Design review of the part built by this model. Coordinates are the model's own, in mm. Give positions to 0.01 mm unless a question says otherwise; leave off trailing zeros. Loops run counter-clockwise (first coordinate to the right, second up) from the corner with the lowest first, then second, coordinate; pieces in that order, holes last. Notation, with made-up numbers: (26, 40.5) -> (42, 40.5) arc R28 ccw to (42, 67.5) -> close; hole circle Ø1 at (76, 62.5). An arc over 180 degrees is marked (long way). Use CSV: the item, a comma, the result in double quotes. Start each with the question number.
Item 1: We need section A-A (x = 279). State the section outline as (y, z) points.
Item 2: Wall thickness on line 1 along X through (y, z) = (-1.25, 0); line 2 along Z through (x, y) = (138.5, 0.9); line 3 along Z through (x, y) = (308.5, 1.7): over which ranges is each line inside the solid? List them lowest first. Write a range as from..to.
Item 3: Clearance check with flat-ended pins moving along their axes: pin 1 (0.6 mm diameter, centred on x = 205, y = 2.5, fed in from +Z); pin 2 (2.5 mm diameter, centred on x = 336.35, z = 0, fed in from -Y); pin 3 (2.5 mm diameter, centred on x = 138, z = -1.5, fed in from +Y). State where each tip first meets the part, or that it passes through.
from build123d import *

# Parameters (mm, degrees)
BOSS_EXTRUDE1_DEPTH = 350
SKETCH6_R           = 1.6
CUT_EXTRUDE1_DEPTH  = 351.117823025


with BuildPart() as part:
    # Sketch5 → Boss-Extrude1 (new body)
    with BuildSketch(Plane(origin=(0, 0, 0), x_dir=(0, 0, -1), z_dir=(1, 0, 0))):
        with BuildLine():
            Line((-8.499999996, -2.75), (8.499999996, -2.75))
            Line((8.499999996, -2.75), (8.499999996, 2.25))
            ThreePointArc((8.499999996, 2.25), (8.353553387, 2.603553391), (7.999999996, 2.75))
            Line((7.999999996, 2.75), (5.299999996, 2.75))
            Line((5.299999996, 2.75), (5.299999996, 1.55))
            Line((5.299999996, 1.55), (7.299999998, 1.55))
            Line((7.299999998, 1.55), (7.299999998, 0.05))
            Line((7.299999998, 0.05), (4.249999998, 0.05))
            Line((4.249999998, 0.05), (3.749999998, -0.45))
            Line((3.749999998, -0.45), (0.499999998, -0.45))
            Line((0.499999998, -0.45), (0, -0.738675133))
            Line((0, -0.738675133), (-0.499999998, -0.45))
            Line((-0.499999998, -0.45), (-3.749999998, -0.45))
            Line((-3.749999998, -0.45), (-4.249999998, 0.05))
            Line((-4.249999998, 0.05), (-7.299999998, 0.05))
            Line((-7.299999998, 0.05), (-7.299999998, 1.55))
            Line((-7.299999998, 1.55), (-5.299999996, 1.55))
            Line((-5.299999996, 1.55), (-5.299999996, 2.75))
            Line((-5.299999996, 2.75), (-7.999999996, 2.75))
            ThreePointArc((-7.999999996, 2.75), (-8.353553387, 2.603553391), (-8.499999996, 2.25))
            Line((-8.499999996, 2.25), (-8.499999996, -2.75))
        make_face()
    extrude(amount=BOSS_EXTRUDE1_DEPTH)

    # Sketch6 → Cut-Extrude1 (cut, through all)
    with BuildSketch(Plane(origin=(0, -0.45, 0), x_dir=(1, 0, 0), z_dir=(0, 1, 0))):
        with Locations(Location((13.647499996, 4e-09, 0), (0, 0, 270))):
            Circle(SKETCH6_R)
        with Locations(Location((3.647499996, 4e-09, 0), (0, 0, 270))):
            Circle(SKETCH6_R)
        with Locations(Location((346.352500004, 4e-09, 0), (0, 0, 270))):
            Circle(SKETCH6_R)
        with Locations(Location((336.352500004, 4e-09, 0), (0, 0, 270))):
            Circle(SKETCH6_R)
    extrude(amount=-CUT_EXTRUDE1_DEPTH, mode=Mode.SUBTRACT)


solid = part.part
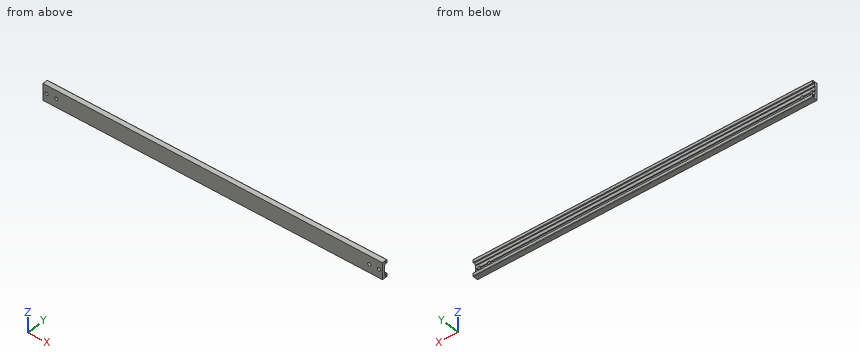
Results found:
1,outline,"(-2.75, -8.5) -> (2.25, -8.5) arc R0.5 ccw to (2.75, -8) -> (2.75, -5.3) -> (1.55, -5.3) -> (1.55, -7.3) -> (0.05, -7.3) -> (0.05, -4.25) -> (-0.45, -3.75) -> (-0.45, -0.5) -> (-0.74, 0) -> (-0.45, 0.5) -> (-0.45, 3.75) -> (0.05, 4.25) -> (0.05, 7.3) -> (1.55, 7.3) -> (1.55, 5.3) -> (2.75, 5.3) -> (2.75, 8) arc R0.5 ccw to (2.25, 8.5) -> (-2.75, 8.5) -> close"
2,line 1,"0..2.05, 5.25..12.05, 15.25..334.75, 337.95..344.75, 347.95..350"
2,line 2,"-8.5..-7.3, 7.3..8.5"
2,line 3,"-8.5..-5.3, 5.3..8.5"
3,pin 1,"z = 8.5"
3,pin 2,"through"
3,pin 3,"y = -0.45"
